Model file for the job. Use its own axes, mm. A direction names the side the tool comes from. Give positions to 0.01 mm unless a question says otherwise; leave off trailing zeros. Write each loop counter-clockwise with the first axis right and the second up, starting at its lowest first coordinate (ties: lowest second). Pieces come first, ordered by that corner, then holes. Notation, with made-up numbers: (86.25, -28.5) - (115.25, -28.5) arc R14 cw to (115.25, -21.5) - close; hole circle Ø3 at (60, 82.25). An arc over 180 degrees is marked (long way). Use CSV: the item, a comma, the result in double quotes.
from build123d import *

# Parameters (mm, degrees)
CYLINDER010_R          = 2.1
CYLINDER010_DEPTH      = 1.5
CYLINDER010_ROLL_ANGLE = 90
CYLINDER008_R          = 2.1
CYLINDER008_DEPTH      = 1.5
CYLINDER008_ROLL_ANGLE = 90
CYLINDER011_R          = 2.1
CYLINDER011_DEPTH      = 1.5
CYLINDER011_ROLL_ANGLE = 90
CYLINDER013_R          = 2.1
CYLINDER013_DEPTH      = 1.5
CYLINDER013_ROLL_ANGLE = 90
CYLINDER012_R          = 2.1
CYLINDER012_DEPTH      = 1.5
CYLINDER012_ROLL_ANGLE = 90
CYLINDER014_R          = 2.1
CYLINDER014_DEPTH      = 1.5
CYLINDER014_ROLL_ANGLE = 90
CYLINDER009_R          = 2.1
CYLINDER009_DEPTH      = 1.5
CYLINDER009_ROLL_ANGLE = 90
CYLINDER_R             = 2.1
CYLINDER_DEPTH         = 1.5
CYLINDER_ROLL_ANGLE    = 90
BOX006_W               = 72
BOX006_H               = 0.75
BOX006_DEPTH           = 10


with BuildPart() as cylinder004:
    # Cylinder010 → Cylinder010 (new body)
    with BuildSketch(Plane.XY):
        Circle(CYLINDER010_R)
    extrude(amount=CYLINDER010_DEPTH)


with BuildPart() as cylinder004_1:
    # Cylinder010 roll: moved
    add(cylinder004.part.rotate(Axis((0, 0, 0), (1, 0, 0)), CYLINDER010_ROLL_ANGLE))


with BuildPart() as cylinder004_2:
    # Cylinder010 placement: moved
    add(cylinder004_1.part.moved(Location((39.72, -0.5, 15.6))))


with BuildPart() as cylinder002:
    # Cylinder008 → Cylinder008 (new body)
    with BuildSketch(Plane.XY):
        Circle(CYLINDER008_R)
    extrude(amount=CYLINDER008_DEPTH)


with BuildPart() as cylinder002_1:
    # Cylinder008 roll: moved
    add(cylinder002.part.rotate(Axis((0, 0, 0), (1, 0, 0)), CYLINDER008_ROLL_ANGLE))


with BuildPart() as cylinder002_2:
    # Cylinder008 placement: moved
    add(cylinder002_1.part.moved(Location((21.72, -0.5, 15.6))))


with BuildPart() as cylinder005:
    # Cylinder011 → Cylinder011 (new body)
    with BuildSketch(Plane.XY):
        Circle(CYLINDER011_R)
    extrude(amount=CYLINDER011_DEPTH)


with BuildPart() as cylinder005_1:
    # Cylinder011 roll: moved
    add(cylinder005.part.rotate(Axis((0, 0, 0), (1, 0, 0)), CYLINDER011_ROLL_ANGLE))


with BuildPart() as cylinder005_2:
    # Cylinder011 placement: moved
    add(cylinder005_1.part.moved(Location((48.72, -0.5, 15.6))))


with BuildPart() as cylinder007:
    # Cylinder013 → Cylinder013 (new body)
    with BuildSketch(Plane.XY):
        Circle(CYLINDER013_R)
    extrude(amount=CYLINDER013_DEPTH)


with BuildPart() as cylinder007_1:
    # Cylinder013 roll: moved
    add(cylinder007.part.rotate(Axis((0, 0, 0), (1, 0, 0)), CYLINDER013_ROLL_ANGLE))


with BuildPart() as cylinder007_2:
    # Cylinder013 placement: moved
    add(cylinder007_1.part.moved(Location((66.72, -0.5, 15.6))))


with BuildPart() as cylinder006:
    # Cylinder012 → Cylinder012 (new body)
    with BuildSketch(Plane.XY):
        Circle(CYLINDER012_R)
    extrude(amount=CYLINDER012_DEPTH)


with BuildPart() as cylinder006_1:
    # Cylinder012 roll: moved
    add(cylinder006.part.rotate(Axis((0, 0, 0), (1, 0, 0)), CYLINDER012_ROLL_ANGLE))


with BuildPart() as cylinder006_2:
    # Cylinder012 placement: moved
    add(cylinder006_1.part.moved(Location((57.72, -0.5, 15.6))))


with BuildPart() as cylinder008:
    # Cylinder014 → Cylinder014 (new body)
    with BuildSketch(Plane.XY):
        Circle(CYLINDER014_R)
    extrude(amount=CYLINDER014_DEPTH)


with BuildPart() as cylinder008_1:
    # Cylinder014 roll: moved
    add(cylinder008.part.rotate(Axis((0, 0, 0), (1, 0, 0)), CYLINDER014_ROLL_ANGLE))


with BuildPart() as cylinder008_2:
    # Cylinder014 placement: moved
    add(cylinder008_1.part.moved(Location((75.72, -0.5, 15.6))))


with BuildPart() as cylinder003:
    # Cylinder009 → Cylinder009 (new body)
    with BuildSketch(Plane.XY):
        Circle(CYLINDER009_R)
    extrude(amount=CYLINDER009_DEPTH)


with BuildPart() as cylinder003_1:
    # Cylinder009 roll: moved
    add(cylinder003.part.rotate(Axis((0, 0, 0), (1, 0, 0)), CYLINDER009_ROLL_ANGLE))


with BuildPart() as cylinder003_2:
    # Cylinder009 placement: moved
    add(cylinder003_1.part.moved(Location((30.72, -0.5, 15.6))))


with BuildPart() as cylinder001:
    # Cylinder → Cylinder (new body)
    with BuildSketch(Plane.XY):
        Circle(CYLINDER_R)
    extrude(amount=CYLINDER_DEPTH)


with BuildPart() as cylinder001_1:
    # Cylinder roll: moved
    add(cylinder001.part.rotate(Axis((0, 0, 0), (1, 0, 0)), CYLINDER_ROLL_ANGLE))


with BuildPart() as cylinder001_2:
    # Cylinder placement: moved
    add(cylinder001_1.part.moved(Location((12.72, -0.5, 15.6))))


with BuildPart() as fusion003005009011:
    # Box006 → Box006 (new body)
    with BuildSketch(Plane(origin=(8.22, -2, 10.6), x_dir=(1, 0, 0), z_dir=(0, 0, 1))):
        with Locations((36, 0.375)):
            Rectangle(BOX006_W, BOX006_H)
    extrude(amount=BOX006_DEPTH)

    # Fusion003005009011: union Cylinder004, Cylinder002, Cylinder005, Cylinder007, Cylinder006, Cylinder008, Cylinder003, Cylinder001
    add(cylinder004_2.part)
    add(cylinder002_2.part)
    add(cylinder005_2.part)
    add(cylinder007_2.part)
    add(cylinder006_2.part)
    add(cylinder008_2.part)
    add(cylinder003_2.part)
    add(cylinder001_2.part)


solid = fusion003005009011.part
(1) Saw through at C-C, the plane x = 49.5. List the corners of the cut face in (y, z).
Checked values:
outline,"(-2, 10.6) - (-1.25, 10.6) - (-1.25, 13.65) - (-0.5, 13.65) - (-0.5, 17.55) - (-1.25, 17.55) - (-1.25, 20.6) - (-2, 20.6) - close"
(2) Wall check: probe 1 along Y at (x, z) = (51, 17.25); probe 2 along Z at (x, y) = (77, -0.55). Give the ranges that are in metal, low to high. Write a range as [from, to].
Checked values:
probe 1,"y = [-2, -1.25]"
probe 2,"z = [13.94, 17.26]"
(3) 3-axis set-ups, long thin cutter, end or side, ignore diameter. For faces 3 (the face through (22, -0.5, 16)), 4 (the face through (77.66, -0.87, 14.8)): which of +Z, -Z, +X, -X, +Y, -Y reach the whole face in a straight line?
Checked values:
face 3,"+Z, -Z, +X, -X, +Y"
face 4,"+Y"
(4) Saw through at B-B, the plane z = 18.75. List the corners of the cut face in (x, y), then the cut area to 3 significant figures.
Checked values:
outline,"(8.22, -2) - (80.22, -2) - (80.22, -1.25) - (8.22, -1.25) - close"
area,"54.0 mm^2"
(5) Flat gauge pin, fed straight in: P1, Ø1.5, axis at x = 70, z = 17, coming from the +Y side. Where does the tip first touch, or does it go through?
Checked values:
P1,"stops at y = -1.25"
(6) Saw through at D-D, the plane x = 17.5. List the corners of the cut face in (y, z).
Checked values:
outline,"(-2, 10.6) - (-1.25, 10.6) - (-1.25, 20.6) - (-2, 20.6) - close"
(7) Pull direction X, two halves, no side cores. Call faces 1 (the face through (23.66, -0.87, 14.8)), 2 (the face through (44, -2, 16)): released by +X, released by -X, zero draft, split by the parting line, or undercut.
Checked values:
face 1,"undercut"
face 2,"zero draft"
(8) Saw through at A-A, the plane x = 39.72. List the corners of the cut face in (y, z), then the cut area to 4 significant figures.
Checked values:
outline,"(-2, 10.6) - (-1.25, 10.6) - (-1.25, 13.5) - (-0.5, 13.5) - (-0.5, 17.7) - (-1.25, 17.7) - (-1.25, 20.6) - (-2, 20.6) - close"
area,"10.65 mm^2"
